```python
from build123d import *

# Parameters (mm, degrees)
SKETCH1_R           = 2.5
SKETCH1_R_2         = 2
BOSS_EXTRUDE1_DEPTH = 4
BOSS_EXTRUDE2_START = 4
SKETCH1_3_R         = 2
BOSS_EXTRUDE2_DEPTH = 10
BOSS_EXTRUDE4_START = 8.9154
SKETCH4_R           = 3.081113055
BOSS_EXTRUDE4_DEPTH = 4
BOSS_EXTRUDE5_DEPTH = 14


with BuildPart() as part:
    # Sketch1 → Boss-Extrude1 (new body)
    with BuildSketch(Plane(origin=(0, 0, 0), x_dir=(1, 0, 0), z_dir=(0, 1, 0))):
        with BuildLine():
            Line((-11.41, 37.5), (11.41, 37.5))
            ThreePointArc((11.41, 37.5), (17.8088531, 35.73800163), (22.403743203, 30.948748641))
            Line((22.403743203, 30.948748641), (39.989594287, -1.551251359))
            ThreePointArc((39.989594287, -1.551251359), (39.733852714, -13.8988531), (28.995851084, -20))
            Line((28.995851084, -20), (-28.995851084, -20))
            ThreePointArc((-28.995851084, -20), (-39.733852714, -13.8988531), (-39.989594287, -1.551251359))
            Line((-39.989594287, -1.551251359), (-22.403743203, 30.948748641))
            ThreePointArc((-22.403743203, 30.948748641), (-17.8088531, 35.73800163), (-11.41, 37.5))
        make_face()
        with Locations((-16.41, 0)):
            Circle(SKETCH1_R, mode=Mode.SUBTRACT)
        with Locations((-11.41, 25)):
            Circle(SKETCH1_R_2, mode=Mode.SUBTRACT)
        with Locations((11.41, 25)):
            Circle(SKETCH1_R_2, mode=Mode.SUBTRACT)
        with Locations((0, 33.5)):
            Circle(SKETCH1_R_2, mode=Mode.SUBTRACT)
        with Locations((31.91, -16.6)):
            Circle(SKETCH1_R_2, mode=Mode.SUBTRACT)
        with Locations((-31.91, -16.6)):
            Circle(SKETCH1_R_2, mode=Mode.SUBTRACT)
    extrude(amount=BOSS_EXTRUDE1_DEPTH)

    # Sketch1_3 → Boss-Extrude2 (add)
    with BuildSketch(Plane(origin=(0, 0, 0), x_dir=(1, 0, 0), z_dir=(0, 1, 0)).offset(BOSS_EXTRUDE2_START)):
        with BuildLine():
            ThreePointArc((-16.41, -20), (-26.18584907, -17.448002034), (-33.466903445, -10.443277496))
            Line((-33.466903445, -10.443277496), (-40.421677434, -12.569565287))
            ThreePointArc((-40.421677434, -12.569565287), (-35.810557017, -17.979016321), (-28.995851084, -20))
            Line((-28.995851084, -20), (-16.41, -20))
        make_face()
        with Locations((-31.91, -16.6)):
            Circle(SKETCH1_3_R, mode=Mode.SUBTRACT)
        with BuildLine():
            ThreePointArc((33.466903445, -10.443277496), (26.18584907, -17.448002034), (16.41, -20))
            Line((16.41, -20), (28.995851084, -20))
            ThreePointArc((28.995851084, -20), (35.810557017, -17.979016321), (40.421677434, -12.569565287))
            Line((40.421677434, -12.569565287), (33.466903445, -10.443277496))
        make_face()
        with Locations((31.91, -16.6)):
            Circle(SKETCH1_3_R, mode=Mode.SUBTRACT)
        with BuildLine():
            Line((6.025107723, 37.5), (-6.025107723, 37.5))
            ThreePointArc((-6.025107723, 37.5), (-1.538984336, 27.943920757), (0, 17.5))
            ThreePointArc((0, 17.5), (1.538984336, 27.943920757), (6.025107723, 37.5))
        make_face()
        with Locations((0, 33.5)):
            Circle(SKETCH1_3_R, mode=Mode.SUBTRACT)
    extrude(amount=BOSS_EXTRUDE2_DEPTH)

    # Sketch4 → Boss-Extrude4 (add)
    with BuildSketch(Plane(origin=(0, 0, 0), x_dir=(0, 0, -1), z_dir=(1, 0, 0)).offset(BOSS_EXTRUDE4_START)):
        Polygon((-20, 0), (-28.99333943, 0), (-60.952260121, 4), (-60.952260121, 14), (-20, 14), align=None)
        with Locations((-49.816366974, 9.411784345)):
            Circle(SKETCH4_R, mode=Mode.SUBTRACT)
    extrude(amount=BOSS_EXTRUDE4_DEPTH)

    # Sketch5 → Boss-Extrude5 (add)
    with BuildSketch(Plane(origin=(0, 14, 0), x_dir=(1, 0, 0), z_dir=(0, 1, 0))):
        Polygon((12.9154, -20), (12.9154, -26.368170387), (25.501140128, -20), align=None)
    extrude(amount=-BOSS_EXTRUDE5_DEPTH)


solid = part.part
```
The model under review builds one solid part; all positions refer to its coordinate system, in mm. A direction names the side the tool comes from. Round coordinates to 2 decimals unless told otherwise and drop trailing zeros. Order: outer loops, then holes, each group sorted by start corner. A loop starts at its lowest first (then second) coordinate and runs counter-clockwise, first axis right, second up. Notation, with made-up numbers: (49, -22) - (92, -22) arc R22 ccw to (92, 2) - close; hole circle Ø7 at (42, -37.5). An arc over 180 degrees is marked (long way). Answer in a Markdown table with one row per item.
(1) Take a section at B-B on z = -33.5. Write out the cut boundary in (x, y), plus the area to 3 significant figures.
Result set:
| item | result |
|---|---|
| outline | (-20.58, 0) - (-2, 0) - (-2, 14) - (-3.73, 14) - (-3.73, 4) - (-20.58, 4) - close; (2, 0) - (20.58, 0) - (20.58, 4) - (3.73, 4) - (3.73, 14) - (2, 14) - close |
| area | 183 mm2 |
(2) Take a section at D-D on y = 2. Write out the cut boundary in (x, z).
Result set:
| item | result |
|---|---|
| outline | (-39.99, 1.55) - (-22.4, -30.95) arc R12.5 ccw to (-11.41, -37.5) - (11.41, -37.5) arc R12.5 ccw to (22.4, -30.95) - (39.99, 1.55) arc R12.5 ccw to (29, 20) - (25.5, 20) - (12.92, 26.37) - (12.92, 44.97) - (8.92, 44.97) - (8.92, 20) - (-29, 20) arc R12.5 ccw to start; hole circle Ø4 at (-31.91, 16.6); hole circle Ø5 at (-16.41, 0); hole circle Ø4 at (-11.41, -25); hole circle Ø4 at (0, -33.5); hole circle Ø4 at (11.41, -25); hole circle Ø4 at (31.91, 16.6) |
(3) Machinability: for faces 5 (the face through (1.496, 8.93, -27.802)), 6 (the face through (17.7, 2, -35.8)), 7 (the face through (-0.434, 6.902, -31.548)), 8 (the face through (-36.896, 8.93, 11.492)), 9 (the face through (-14.5, 3.8, 20)), which of the approach directions +Z, -Z, +X, -X, +Y, -Y give a long, thin tool a straight path to every point of the face, cutting with its end or side? Answer none if there is none.
Result set:
| item | result |
|---|---|
| face 5 | +Z, +X, +Y |
| face 6 | -Z, +X, +Y, -Y |
| face 7 | +Y, -Y |
| face 8 | -Z, -X, +Y |
| face 9 | +Z, -X, +Y, -Y |
(4) Take a section at A-A on y = 11.25. Write out the cut boundary in (x, z).
Result set:
| item | result |
|---|---|
| outline | (-40.42, 12.57) - (-33.47, 10.44) arc R20 cw to (-16.41, 20) - (-29, 20) arc R12.5 ccw to start; (-6.03, -37.5) - (6.03, -37.5) arc R36.21 cw to (0, -17.5) arc R36.21 cw to start; (8.92, 20) - (16.41, 20) arc R20 cw to (33.47, 10.44) - (40.42, 12.57) arc R12.5 ccw to (29, 20) - (25.5, 20) - (12.92, 26.37) - (12.92, 47.34) - (8.92, 47.34) - close; (8.92, 52.29) - (12.92, 52.29) - (12.92, 60.95) - (8.92, 60.95) - close; hole circle Ø4 at (-31.91, 16.6); hole circle Ø4 at (0, -33.5); hole circle Ø4 at (31.91, 16.6) |
(5) For line 1 (X direction, y = 8.5, z = 16.6); line 2 (X direction, y = 11.25, z = 15.5); line 3 (X direction, y = 4.5, z = 56.5), list the stretches that pass through material, from the lowest coordinate up. Write a range as from..to.
Result set:
| item | result |
|---|---|
| line 1 | x = -37.57..-33.91, -29.91..-27.57, 27.57..29.91, 33.91..37.57 |
| line 2 | x = -38.6..-33.58, -30.24..-29.05, 29.05..30.24, 33.58..38.6 |
| line 3 | x = 8.92..12.92 |
(6) Take a section at C-C on x = -31.91. Write out the cut boundary in (y, z).
Result set:
| item | result |
|---|---|
| outline | (0, -13.38) - (4, -13.38) - (4, 12.64) - (14, 12.64) - (14, 14.6) - (0, 14.6) - close; (0, 18.6) - (14, 18.6) - (14, 19.66) - (0, 19.66) - close |
(7) Mouldability with a two-part tool opening along X and no side actions: class faces 1 (the face through (2, 14, -32)), 2 (the face through (-12.997, 1.972, -23.783)), 3 (the face through (8.915, 7, 40)), 4 (the face through (-16.95, 1.97, 2.44)) as released by +X, released by -X, zero draft, split by the parting line, or undercut.
Result set:
| item | result |
|---|---|
| face 1 | zero draft |
| face 2 | undercut |
| face 3 | released by -X |
| face 4 | undercut |
(8) Clearance check with flat-ended pins moving along their axes: P1, Ø6, axis at x = 13, y = 9, coming from the -Z side; P2, Ø8, axis at x = 30, y = 2, coming from the +Z side; P3, Ø2.5, axis at x = -31.91, z = 16.6, coming from the -Y side; P4, Ø6.5, axis at x = 11.41, z = -25, coming from the +Y side. State where each tip first meets the part, or that it passes through.
Result set:
| item | result |
|---|---|
| P1 | stops at z = 20 |
| P2 | stops at z = 20 |
| P3 | passes through |
| P4 | stops at y = 4 |
